For this review, use the dimensioned drawing (mm, ordinates from the lowest corner) and the shaded views. A direction names the side the tool comes from. Coordinates: 2 decimals unless noted, no trailing zeros. Order: outer loops, then holes, each group sorted by start corner. A loop starts at its lowest first (then second) coordinate and runs counter-clockwise, first axis right, second up. Notation, with made-up numbers: M -31,68.5 L -13,68.5 A14 cw -13,94.5 Z; hole C -38.5,57.5 d3. An arc over 180 degrees is marked long. Write each question's results on one line, items separated by ' | '.
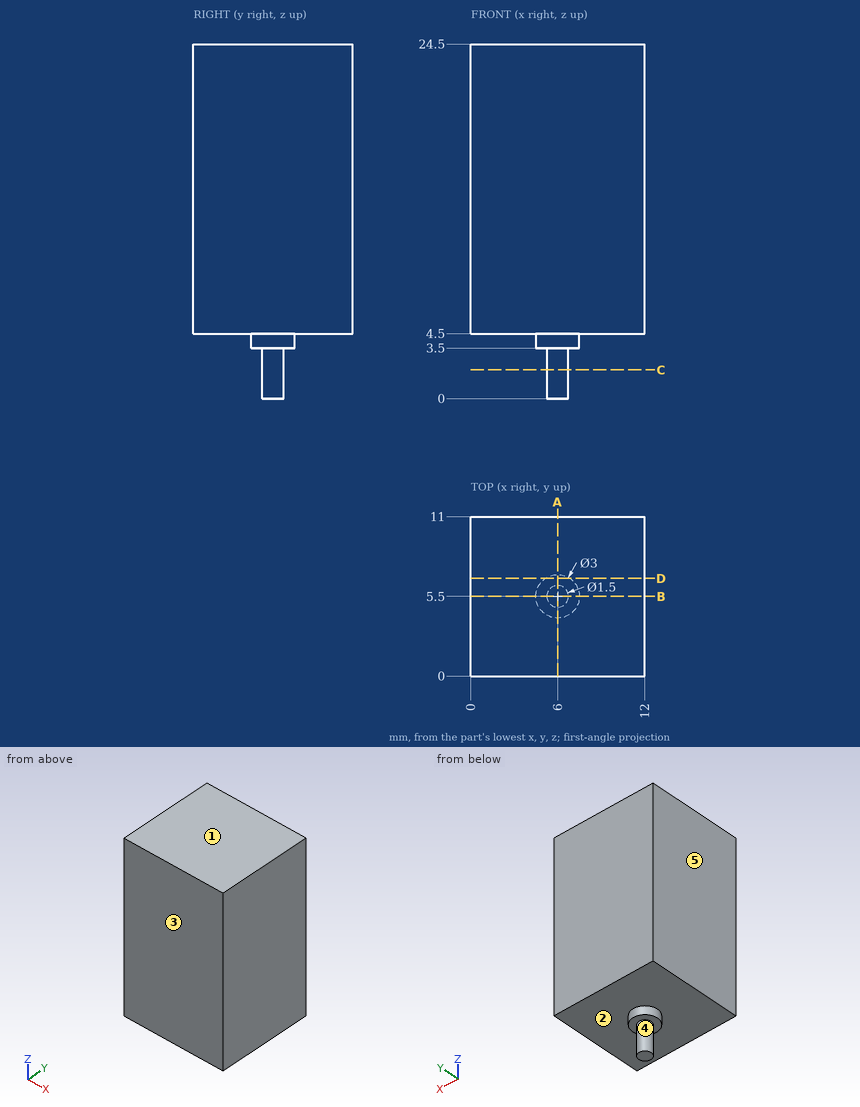
1) Take a section at A-A on x = 6. State the section outline as (y, z) points.
Solutions:
outline: M 0,4.5 L 4,4.5 L 4,3.5 L 4.75,3.5 L 4.75,0 L 6.25,0 L 6.25,3.5 L 7,3.5 L 7,4.5 L 11,4.5 L 11,24.5 L 0,24.5 Z
2) The part is to be moulded in two halves that separate along Z. For the marked faces 1, 2 and 3, say which applies: pulls with the +Z half, pulls with the -Z half, needs draft (parallel to the pull), parting line crosses it, or undercut.
Solutions:
face 1: pulls with the +Z half | face 2: pulls with the -Z half | face 3: needs draft
3) Take a section at B-B on y = 5.5. State the section outline as (x, z) points.
Solutions:
outline: M 0,4.5 L 4.5,4.5 L 4.5,3.5 L 5.25,3.5 L 5.25,0 L 6.75,0 L 6.75,3.5 L 7.5,3.5 L 7.5,4.5 L 12,4.5 L 12,24.5 L 0,24.5 Z
4) To check wall thickness, follow line 1 along Z through (x, y) = (2.75, 4.5). State the ranges of the line that lie inside material, in increasing order.
Solutions:
line 1: 4.5 to 24.5
5) Take a section at C-C on z = 2. State the section outline as (x, y) points.
Solutions:
outline: C 6,5.5 d1.5
6) For the marked faces 4 and 5, list the 3-axis set-ups (+Z, -Z, +X, -X, +Y, -Y) from which the entire face can be reached by the end or side of a thin tool; tool diameter is ignored.
Solutions:
face 4: -Z | face 5: +Z, -Z, -X, +Y, -Y
7) Take a section at D-D on y = 6.75. State the section outline as (x, z) points.
Solutions:
outline: M 0,4.5 L 5.17,4.5 L 5.17,3.5 L 6.83,3.5 L 6.83,4.5 L 12,4.5 L 12,24.5 L 0,24.5 Z
